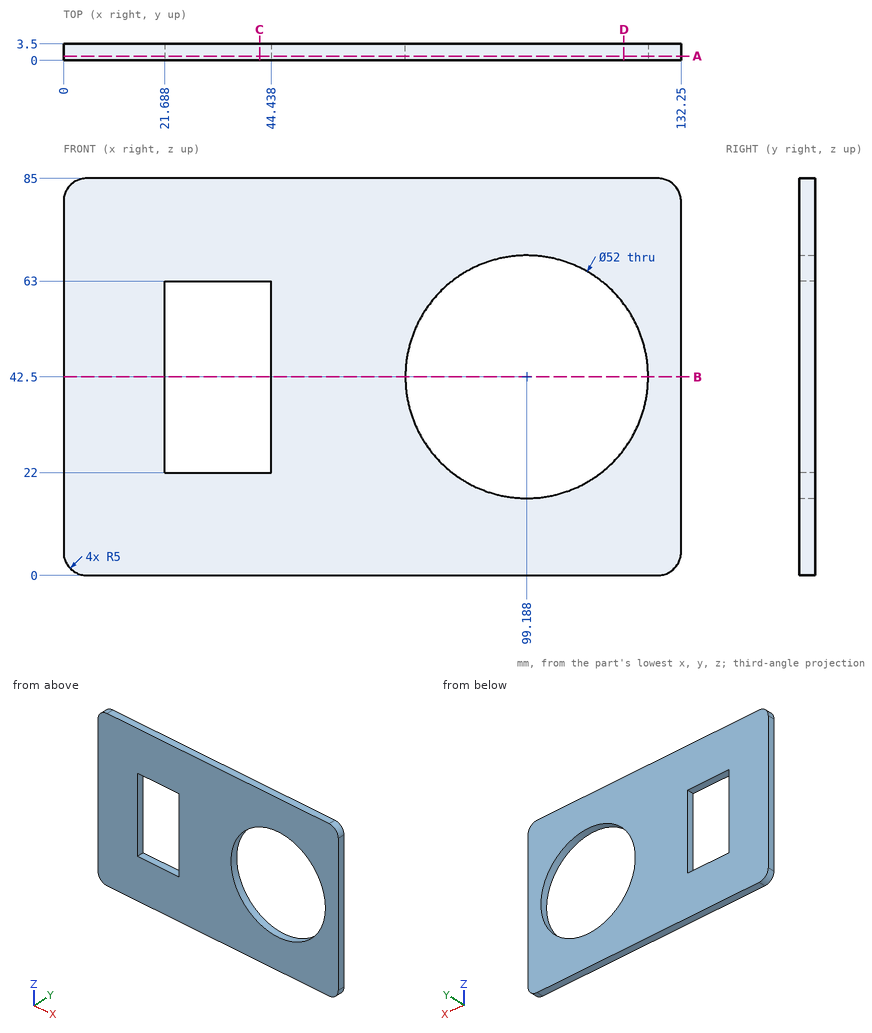
The drawing under review shows one solid part. Ordinate dimensions are in mm from its lowest x, y, z. Give positions to 0.01 mm unless a question says otherwise; leave off trailing zeros. Write each loop counter-clockwise with the first axis right and the second up, starting at its lowest first coordinate (ties: lowest second). Pieces come first, ordered by that corner, then holes. Notation, with made-up numbers: (82, 77) -> (101, 77) arc R18 cw to (101, 87) -> close; hole circle Ø11 at (-38.75, -32). An arc over 180 degrees is marked (long way). Use CSV: the item, a comma, the result in double quotes.
Q1. Take a section at D-D, the plane x = 120. Write out the cut boundary in (y, z).
Conclusion:
outline,"(0, 0) -> (3.5, 0) -> (3.5, 26.92) -> (0, 26.92) -> close; (0, 58.08) -> (3.5, 58.08) -> (3.5, 85) -> (0, 85) -> close"
Q2. Take a section at C-C, the plane x = 42. Write out the cut boundary in (y, z), then the cut area to 3 significant figures.
Conclusion:
outline,"(0, 0) -> (3.5, 0) -> (3.5, 22) -> (0, 22) -> close; (0, 63) -> (3.5, 63) -> (3.5, 85) -> (0, 85) -> close"
area,"154 mm2"
Q3. Take a section at A-A, the plane y = 0.9. Write out the cut boundary in (x, z).
Conclusion:
outline,"(0, 5) arc R5 ccw to (5, 0) -> (127.25, 0) arc R5 ccw to (132.25, 5) -> (132.25, 80) arc R5 ccw to (127.25, 85) -> (5, 85) arc R5 ccw to (0, 80) -> close; hole (21.69, 22) -> (44.44, 22) -> (44.44, 63) -> (21.69, 63) -> close; hole circle Ø52 at (99.19, 42.5)"
Q4. To check wall thickness, follow probe 1 along X at (y, z) = (0.65, 30.5); probe 2 along X at (y, z) = (3.1, 46.5); probe 3 along Z at (x, y) = (36, 2.9). State the ranges of each line that lie inside material, in increasing order. Write a range as [from, to].
Conclusion:
probe 1,"[0, 21.69], [44.44, 76.12], [122.25, 132.25]"
probe 2,"[0, 21.69], [44.44, 73.5], [124.88, 132.25]"
probe 3,"[0, 22], [63, 85]"
Q5. For P1, Ø6, axis at x = 86.5, z = 60.5, coming from the -Y side, flat-tipped, find the tip position at first contact; note if it passes through.
Conclusion:
P1,"through"
Q6. Take a section at B-B, the plane z = 42.5. Write out the cut boundary in (x, y).
Conclusion:
outline,"(0, 0) -> (21.69, 0) -> (21.69, 3.5) -> (0, 3.5) -> close; (44.44, 0) -> (73.19, 0) -> (73.19, 3.5) -> (44.44, 3.5) -> close; (125.19, 0) -> (132.25, 0) -> (132.25, 3.5) -> (125.19, 3.5) -> close"
